Autodesk Inventor part; units mm, degrees
ref_plane "YZ Plane" through (0, 0, 0) normal (1, 0, 0) x (0, 1, 0)
ref_plane "XZ Plane" through (0, 0, 0) normal (0, 1, 0) x (-1, 0, 0)
ref_plane "XY Plane" through (0, 0, 0) normal (0, 0, 1) x (1, 0, 0)
sketch "Esboço1" plane through (0, 0, 0) normal (0, 0, 1) x (1, 0, 0)
  arc A0 (5, -8.6603) -> (-5, -8.6603) centre (0, 0) ccw
  line L0 (0, 0) -> (3, 0)
  line L1 (0, 0) -> (3, 0) construction
  line L2 (-2.5, -4.3301) -> (-5, -8.6603)
  line L3 (2.5, -4.3301) -> (5, -8.6603)
  line L4 (-2.5, 4.3301) -> (-3, 5.1962)
  line L5 (2.5, 4.3301) -> (3, 5.1962)
  arc A1 (-3, 5.1962) -> (-5.7956, -1.5529) centre (0, 0) ccw
  arc A2 (5.7956, -1.5529) -> (3, 5.1962) centre (0, 0) ccw
  arc A3 (-4.8296, -1.2941) -> (-2.5, -4.3301) centre (0, 0) ccw
  arc A4 (2.5, -4.3301) -> (4.8296, -1.2941) centre (0, 0) ccw
  arc A5 (2.5, 4.3301) -> (-2.5, 4.3301) centre (0, 0) ccw
  line L6 (-4.8296, -1.2941) -> (-5.7956, -1.5529)
  line L7 (4.8296, -1.2941) -> (5.7956, -1.5529)
  dimension "d3" = 3
  dimension "d4" = 0
  dimension "d5" = 60
  dimension "d6" = 60
  dimension "d9" = 45
  dimension "d10" = 45
  dimension "d11" = 5
  dimension "d12" = 5
  dimension "d13" = 6
  dimension "d14" = 6
  dimension "d15" = 5
  dimension "d20" = 4
extrude "Placa1" add sketch "Esboço1" along normal blind 1
fillet "Arredondamento de canto1" radius 1 4 edges at (-2.5, -4.3301, 0.5) (-5, -8.6603, 0.5) (5, -8.6603, 0.5) (2.5, -4.3301, 0.5)
fillet "Arredondamento de canto2" radius 0.35 8 edges at (-4.8296, -1.2941, 0.5) (-5.7956, -1.5529, 0.5) (-2.5, 4.3301, 0.5) (-3, 5.1962, 0.5) (2.5, 4.3301, 0.5) (3, 5.1962, 0.5) (5.7956, -1.5529, 0.5) (4.8296, -1.2941, 0.5)
equation "\"d12\" = d15"
equation "\"d13\" = d14"
equation "\"d15\" = d11"
equation "\"Raio_dobra\" = Espessura"
equation "\"Largura_alívio_de_dobra\" = Espessura"
equation "\"Profundidade_alívio_de_dobra\" = 0.5 * Espessura"
equation "\"Tamanho_alívio_de_dobra\" = 4 * Espessura"
equation "\"Remanescente_mínimo\" = 2 * Espessura"
equation "\"Raiodetransição\" = Raio_dobra"
equation "\"Tamanho_de_raio_de_Jacobi\" = Raio_dobra"
equation "\"TamanhoFolga\" = Espessura"
equation "\"d8\" = d7"
equation "\"d17\" = Raio_dobra"
properties part number "anel_elastico" material "Padrão"
Can you work these out from the model? Positions are in its coordinate system, mm. A direction names the side the tool comes from. Round coordinates to 2 decimals unless told otherwise and drop trailing zeros. Loops run counter-clockwise (first coordinate to the right, second up) from the corner with the lowest first, then second, coordinate; pieces in that order, holes last.
Item 1: Suppose I cut it at D-D, the plane y = -5.5. Write out the boundary of the cut face in (x, z).
Item 2: Suppose I cut it at A-A, the plane y = 0. Write out the boundary of the cut face in (x, z).
Item 3: Please list where these lines run through material, in increasing order: L1, parallel to Y at x = -8, z = 0.7; L2, parallel to X at y = -6.25, z = 0.2; L3, parallel to X at y = 2.75, z = 0.8.
Item 4: Suppose I cut it at B-B, the plane z = 0.4. Write out the boundary of the cut face in (x, y).
Item 5: Which directions (+Z, -Z, +X, -X, +Y, -Y) give clear straight access to the entire face, cutting with the end or side of a thin tool? Please do faces 5 (the flat face through (-3.704, -6.416, 0.493)), 6 (the flat face through (-2, 5, 0)), 7 (the cylindrical face through (-2.838, -4.456, 0.507)).
Item 6: If we mould it in two halves opening along Y, with no side actions, what happens to faces 1 (the cylindrical face through (-4.11, -2.85, 0.49)), 2 (the flat face through (-2, 5, 1)), 3 (the flat face through (3.704, -6.416, 0.493)), 4 (the cylindrical face through (2.84, -4.44, 0.51))? For each: +Y half, -Y half, draft (parallel to the pull), parting line (faces both ways), or undercut.
Item 7: Suppose I cut it at C-C, the plane x = 0. Write out the boundary of the cut face in (y, z).
Reported:
1. outline: (-8.35, 0) - (-3.18, 0) - (-3.18, 1) - (-8.35, 1) - close; (3.18, 0) - (8.35, 0) - (8.35, 1) - (3.18, 1) - close
2. outline: (-10, 0) - (-6, 0) - (-6, 1) - (-10, 1) - close; (6, 0) - (10, 0) - (10, 1) - (6, 1) - close
3. L1: y = -6 to 6
3. L2: x = -7.81 to -3.61, 3.61 to 7.81
3. L3: x = -9.61 to -5.33, 5.33 to 9.61
4. outline: (-5.93, -8.05) arc R1 ccw to (-4.47, -7.75) - (-2.96, -5.12) arc R1 ccw to (-3.19, -3.85) arc R5 cw to (-4.73, -1.61) arc R0.35 ccw to (-5.16, -1.38) - (-5.45, -1.46) arc R0.35 cw to (-5.88, -1.19) arc R6 cw to (-3.32, 5) arc R0.35 cw to (-2.82, 4.88) - (-2.67, 4.62) arc R0.35 ccw to (-2.21, 4.48) arc R5 cw to (2.21, 4.48) arc R0.35 ccw to (2.67, 4.62) - (2.82, 4.88) arc R0.35 cw to (3.32, 5) arc R6 cw to (5.88, -1.19) arc R0.35 cw to (5.45, -1.46) - (5.16, -1.38) arc R0.35 ccw to (4.73, -1.61) arc R5 cw to (3.19, -3.85) arc R1 ccw to (2.96, -5.12) - (4.47, -7.75) arc R1 ccw to (5.93, -8.05) arc R10 ccw (long way) to start
5. face 5: +Z, -Z, -Y
5. face 6: -Z, +X, -X, +Y, -Y
5. face 7: +Z, -Z
6. face 1: undercut
6. face 2: draft
6. face 3: -Y half
6. face 4: undercut
7. outline: (5, 0) - (10, 0) - (10, 1) - (5, 1) - close
